from build123d import *

# Parameters (mm, degrees)
CROQUIS1_W                   = 10
CROQUIS1_H                   = 10
SALIENTE_EXTRUIR1_DEPTH      = 77.5
TALADRO_DE_MARGEN_PARA_M31_D = 3.75
CORTAR_EXTRUIR1_DEPTH        = 3
TALADRO_DE_MARGEN_PARA_M32_D = 3.75
CORTAR_EXTRUIR2_DEPTH        = 3
CORTAR_EXTRUIR3_DEPTH        = 3.2
MATRIZL1_COUNT               = 3
MATRIZL1_PITCH               = 30
MATRIZL1_COL_COUNT           = 2
MATRIZL1_COL_PITCH           = 30


with BuildPart() as part:
    # Croquis1 → Saliente-Extruir1 (new body, symmetric)
    with BuildSketch(Plane.XY):
        Rectangle(CROQUIS1_W, CROQUIS1_H)
    extrude(amount=SALIENTE_EXTRUIR1_DEPTH, both=True)

    # Taladro de margen para M31 (through all)
    with Locations(Plane(origin=(0, 5, 0), x_dir=(1, 0, 0), z_dir=(0, 1, 0))):
        with Locations((0, -60), (0, 0), (0, 60)):
            Hole(TALADRO_DE_MARGEN_PARA_M31_D / 2)

    # Croquis7 → Cortar-Extruir1 (cut)
    with BuildSketch(Plane.XZ.offset(5)):
        Polygon((2.771281292, -58.4), (0, -56.8), (-2.771281292, -58.4), (-2.771281292, -61.6), (0, -63.2), (2.771281292, -61.6), align=None)
        Polygon((2.771281292, -1.6), (2.771281292, 1.6), (0, 3.2), (-2.771281292, 1.6), (-2.771281292, -1.6), (0, -3.2), align=None)
        Polygon((2.771281292, 58.4), (2.771281292, 61.6), (0, 63.2), (-2.771281292, 61.6), (-2.771281292, 58.4), (0, 56.8), align=None)
    extrude(amount=-CORTAR_EXTRUIR1_DEPTH, mode=Mode.SUBTRACT)

    # Taladro de margen para M32 (through all)
    with Locations(Plane.ZY.offset(5)):
        with Locations((-30, 0), (30, 0)):
            Hole(TALADRO_DE_MARGEN_PARA_M32_D / 2)

    # Croquis10 → Cortar-Extruir2 (cut)
    with BuildSketch(Plane.ZY.offset(5)):
        Polygon((-28.4, -2.771281292), (-26.8, 0), (-28.4, 2.771281292), (-31.6, 2.771281292), (-33.2, 0), (-31.6, -2.771281292), align=None)
        Polygon((31.6, -2.771281292), (33.2, 0), (31.6, 2.771281292), (28.4, 2.771281292), (26.8, 0), (28.4, -2.771281292), align=None)
    extrude(amount=-CORTAR_EXTRUIR2_DEPTH, mode=Mode.SUBTRACT)

    # Croquis13 → Taladro de margen para M33 (revolve, cut)
    with BuildSketch(Plane(origin=(-5, 0, -15), x_dir=(0, 0, 1), z_dir=(0, 1, 0))):
        Polygon((0, 0), (0, 7.126613661), (1.875, 6), (1.875, 0), align=None)
    taladro_de_margen_para_m33 = revolve(axis=Axis((-11.35, 0, -15), (1, 0, 0)), mode=Mode.SUBTRACT)

    # Croquis15 → Cortar-Extruir3 (cut)
    with BuildSketch(Plane.ZY):
        Polygon((-18.6, -5), (-11.4, -5), (-11.4, 0), (-13.2, -3.117691454), (-16.8, -3.117691454), (-18.6, 0), align=None)
        Polygon((-16.8, -3.117691454), (-13.2, -3.117691454), (-11.4, 0), (-13.2, 3.117691454), (-16.8, 3.117691454), (-18.6, 0), align=None)
    cortar_extruir3 = extrude(amount=-CORTAR_EXTRUIR3_DEPTH, mode=Mode.SUBTRACT)

    # MatrizL1: Taladro de margen para M33, Cortar-Extruir3 ×3
    with Locations(*[(0, 0, i * MATRIZL1_PITCH) for i in range(1, MATRIZL1_COUNT)]):
        add(taladro_de_margen_para_m33, mode=Mode.SUBTRACT)
        add(cortar_extruir3, mode=Mode.SUBTRACT)

    # MatrizL1 col: Taladro de margen para M33, Cortar-Extruir3 ×2
    with Locations(*[(0, 0, -i * MATRIZL1_COL_PITCH) for i in range(1, MATRIZL1_COL_COUNT)]):
        add(taladro_de_margen_para_m33, mode=Mode.SUBTRACT)
        add(cortar_extruir3, mode=Mode.SUBTRACT)


solid = part.part
Can you work these out from the model? Positions are in its coordinate system, mm. A direction names the side the tool comes from. Give positions to 0.01 mm unless a question says otherwise; leave off trailing zeros. Loops run counter-clockwise (first coordinate to the right, second up) from the corner with the lowest first, then second, coordinate; pieces in that order, holes last. Notation, with made-up numbers: (17, 38.25) - (58, 38.25) arc R31 cw to (58, 74.25) - close; hole circle Ø4 at (-36, -24). An arc over 180 degrees is marked (long way). Return JSON: item names as keys, results as strings.
1. I want a section at B-B on z = -30. Please give me the cut outline in (x, y) (3 decimals), and give its area (3 significant figures).
Output values:
{"outline": "(-5, -5) - (5, -5) - (5, -1.875) - (-2, -1.875) - (-2, -2.771) - (-5, -2.771) - close; (-5, 2.771) - (-2, 2.771) - (-2, 1.875) - (5, 1.875) - (5, 5) - (-5, 5) - close", "area": "57.1 mm²"}
2. I'm going to push flat-ended pins straight in: pin 1 Ø1.7 at (x, z) = (0, -60) entering from -Y; pin 2 Ø4.5 at (y, z) = (-1.5, 30) entering from -X. Where does each tip first touch, or does it pass through?
Output values:
{"pin 1": "passes through", "pin 2": "stops at x = -5"}
3. If I drill on line 1 (Z direction, x = -1, y = 2.75); line 2 (Y direction, x = 2.25, z = -30) (3 decimals); line 3 (Y direction, x = -1.25, z = 31), over which ranges is the centre line in solid material (lowest first)?
Output values:
{"line 1": "z = -77.5 to -61.59, -58.41 to -1.59, 1.59 to 58.41, 61.59 to 77.5", "line 2": "y = -5 to -1.875, 1.875 to 5", "line 3": "y = -5 to -1.59, 1.59 to 5"}
4. I want a section at A-A on z = 45. Please give me the cut outline in (x, y) (3 decimals).
Output values:
{"outline": "(-5, -5) - (0, -5) - (0, -1.875) - (-5, -1.875) - close; (-5, 1.875) - (0, 1.875) - (0, 3.118) - (3.2, 3.118) - (3.2, -5) - (5, -5) - (5, 5) - (-5, 5) - close"}
5. For faces 1 (the face through (-3.521, 1.405, -32.389)), 2 (the face through (0.24, 1.45, -61.86)), 3 (the face through (1.58, 1.54, 47.71)), which set-ups out of +Z, -Z, +X, -X, +Y, -Y let a thin tool reach every point of the face, with its end or its side?
Output values:
{"face 1": "-X", "face 2": "+Y, -Y", "face 3": "-Y"}
